Model file for the job. Use its own axes, mm. A direction names the side the tool comes from. Coordinates: 2 decimals unless noted, no trailing zeros. Write each loop counter-clockwise with the first axis right and the second up, starting at its lowest first coordinate (ties: lowest second). Pieces come first, ordered by that corner, then holes.
Q1. Band-saw the part on D-D, the plane z = 36.75. State how many separate pieces and enclosed holes the cut face has, plus the area to 3 significant figures.
Q2. Band-saw the part on C-C, the plane y = 8. Write the cut outline in (x, z), plus the area to 3 significant figures.
Q3. Band-saw the part on A-A, the plane x = 0. Write the cut outline in (y, z).
Q4. Band-saw the part on B-B, the plane x = -62. Write the cut outline in (y, z).
Q5. Pull direction X, two halves, no side cores. Call faces 1 (the flat face through (-74, -46.75, 36)), 2 (the flat face through (16.448, -60.842, 36.236)), 3 (the flat face through (26.4, 19.03, 36.24)), 4 (the flat face through (-16.552, -61.158, 36.236)): released by +X, released by -X, zero draft, split by the parting line, or undercut.
Q6. Pin check, flat tips, straight feed: P1, Ø7.5, axis at x = 34.5, z = 49.5, coming from the +Y side; P2, Ø11, axis at x = -0.5, z = 36.5, coming from the +Y side; P3, Ø1.5, axis at y = -33, z = 22.5, coming from the -X side; P4, Ø20, axis at y = -10, z = 39, coming from the -X side. Stop position of each tip, or through.
Q7. Drill centre lines: probe 1 along Y at (x, z) = (2, 20); probe 2 along Y at (x, z) = (33.5, 45.5); probe 3 along X at (y, z) = (-42, 8). Where is each one in solid material? Low to high.
Q8. Which spindle directions (+Z, -Z, +X, -X, +Y, -Y) get a long thin tool onto all of the face, cutting with end or side? Do faces 5 (the flat face through (73, -46.75, 36)), 6 (the flat face through (8, -22, 73.5)), 7 (the flat face through (-10.25, 0, 36)). Say none if no direction does.
from build123d import *

# Parameters (mm, degrees)
SKETCH1_W           = 20.5
SKETCH1_H           = 20.5
BOSS_EXTRUDE1_DEPTH = 73.5
SKETCH2_R           = 2.75
CUT_EXTRUDE1_DEPTH  = 33.5
SKETCH3_R           = 5
CUT_EXTRUDE2_DEPTH  = 6.5


with BuildPart() as part:
    # Sketch1 → Boss-Extrude1 (new body)
    with BuildSketch(Plane.XY):
        Polygon((-87.236832981, -46.75), (-59.907888654, -46.75), (-39.429270613, 14.685854123), (-13.736832981, 23.25), (13.736832981, 23.25), (39.429270613, 14.685854123), (59.907888654, -46.75), (87.236832981, -46.75), (96.736832981, -75.25), (-96.736832981, -75.25), align=None)
        Polygon((-13.25, 20.25), (-13.25, -20.25), (-35.75, -12.75), (-35.75, 12.75), align=None, mode=Mode.SUBTRACT)
        Rectangle(SKETCH1_W, SKETCH1_H, mode=Mode.SUBTRACT)
        Polygon((13.25, -20.25), (35.75, -12.75), (35.75, 12.75), (13.25, 20.25), align=None, mode=Mode.SUBTRACT)
        Polygon((-12.75, -49.75), (12.75, -49.75), (20.25, -72.25), (-20.25, -72.25), align=None, mode=Mode.SUBTRACT)
        Polygon((15.91227766, -49.75), (23.41227766, -72.25), (48.91227766, -72.25), (56.41227766, -49.75), align=None, mode=Mode.SUBTRACT)
        Polygon((-48.91227766, -72.25), (-56.41227766, -49.75), (-15.91227766, -49.75), (-23.41227766, -72.25), align=None, mode=Mode.SUBTRACT)
        Polygon((59.57455532, -49.75), (52.07455532, -72.25), (92.57455532, -72.25), (85.07455532, -49.75), align=None, mode=Mode.SUBTRACT)
        Polygon((-92.57455532, -72.25), (-85.07455532, -49.75), (-59.57455532, -49.75), (-52.07455532, -72.25), align=None, mode=Mode.SUBTRACT)
        Polygon((48.91227766, -23.25), (56.41227766, -45.75), (15.91227766, -45.75), (23.41227766, -23.25), align=None, mode=Mode.SUBTRACT)
        Polygon((20.25, -23.25), (-20.25, -23.25), (-12.75, -45.75), (12.75, -45.75), align=None, mode=Mode.SUBTRACT)
        Polygon((-23.41227766, -23.25), (-48.91227766, -23.25), (-56.41227766, -45.75), (-15.91227766, -45.75), align=None, mode=Mode.SUBTRACT)
    extrude(amount=BOSS_EXTRUDE1_DEPTH)

    # Sketch2 → Cut-Extrude1 (cut)
    with BuildSketch(Plane(origin=(0, 23.25, 0), x_dir=(1, 0, 0), z_dir=(0, 1, 0))):
        with Locations(Location((0, -36.75, 0), (0, 0, 270))):
            Circle(SKETCH2_R)
    extrude(amount=-CUT_EXTRUDE1_DEPTH, mode=Mode.SUBTRACT)

    # Sketch3 → Cut-Extrude2 (cut)
    with BuildSketch(Plane(origin=(0, 23.25, 0), x_dir=(1, 0, 0), z_dir=(0, 1, 0))):
        with Locations(Location((0, -36.75, 0), (0, 0, 270))):
            Circle(SKETCH3_R)
    extrude(amount=-CUT_EXTRUDE2_DEPTH, mode=Mode.SUBTRACT)


solid = part.part
Answer sheet:
1. separate pieces: 1
1. enclosed holes: 10
1. area: 3,860 mm2
2. outline: (-41.66, 0) - (-35.75, 0) - (-35.75, 73.5) - (-41.66, 73.5) - close; (-13.25, 0) - (-10.25, 0) - (-10.25, 73.5) - (-13.25, 73.5) - close; (10.25, 0) - (13.25, 0) - (13.25, 73.5) - (10.25, 73.5) - close; (35.75, 0) - (41.66, 0) - (41.66, 73.5) - (35.75, 73.5) - close
2. area: 1,310 mm2
3. outline: (-75.25, 0) - (-72.25, 0) - (-72.25, 73.5) - (-75.25, 73.5) - close; (-49.75, 0) - (-45.75, 0) - (-45.75, 73.5) - (-49.75, 73.5) - close; (-23.25, 0) - (-10.25, 0) - (-10.25, 73.5) - (-23.25, 73.5) - close; (10.25, 0) - (23.25, 0) - (23.25, 31.75) - (16.75, 31.75) - (16.75, 34) - (10.25, 34) - close; (10.25, 39.5) - (16.75, 39.5) - (16.75, 41.75) - (23.25, 41.75) - (23.25, 73.5) - (10.25, 73.5) - close
4. outline: (-75.25, 0) - (-72.25, 0) - (-72.25, 73.5) - (-75.25, 73.5) - close; (-49.75, 0) - (-46.75, 0) - (-46.75, 73.5) - (-49.75, 73.5) - close
5. face 1: zero draft
5. face 2: undercut
5. face 3: released by +X
5. face 4: undercut
6. P1: stops at y = 17.58
6. P2: stops at y = 23.25
6. P3: stops at x = -55.57
6. P4: stops at x = -50.99
7. probe 1: y = -75.25 to -72.25, -49.75 to -45.75, -23.25 to -10.25, 10.25 to 23.25
7. probe 2: y = -75.25 to -72.25, -49.75 to -45.75, -23.25 to -13.5, 13.5 to 16.66
7. probe 3: x = -58.32 to -55.16, -17.16 to -14, 14 to 17.16, 55.16 to 58.32
8. face 5: +Z, -Z, +X, +Y
8. face 6: +Z, +X, -X, +Y, -Y
8. face 7: +Z, -Z
